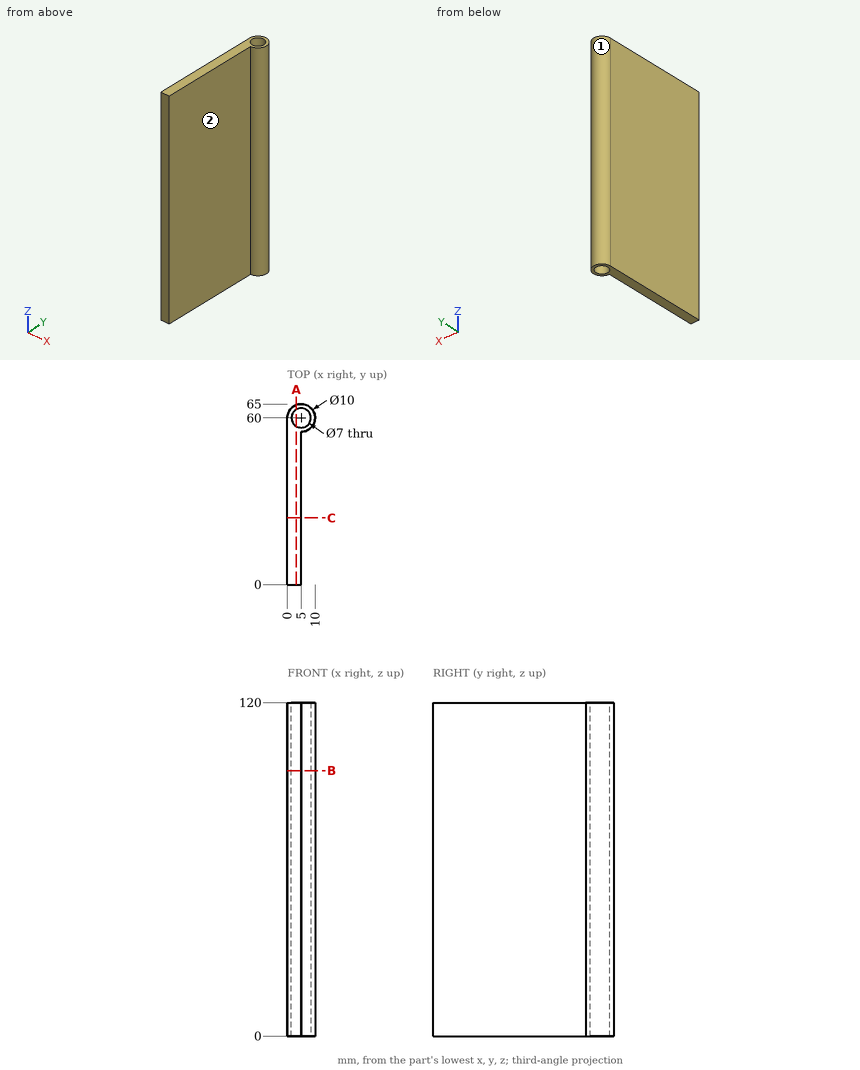
Could you check a few things on this drawing? It's one solid part, dimensions in mm from its lowest x, y, z. A direction names the side the tool comes from. Round coordinates to 2 decimals unless told otherwise and drop trailing zeros. Loops run counter-clockwise (first coordinate to the right, second up) from the corner with the lowest first, then second, coordinate; pieces in that order, holes last. Notation, with made-up numbers: M -29.5,77 L 27.5,77 A17 ccw 27.5,96 Z; hole C 0.5,-28.5 d1. An arc over 180 degrees is marked long. Write item = value, one per line. Start each with the question number.
(1) Which directions (+Z, -Z, +X, -X, +Y, -Y) give clear straight access to the entire face, cutting with the end or side of a thin tool? Please do the marked faces 1 and 2.
(2) I'm going to push a flat-ended pin straight in: P1, Ø6, axis at y = 10.5, z = 35.5, coming from the -X side. Where does the tip first touch, or does it pass through?
(3) Suppose I cut it at A-A on x = 3.25. Write out the boundary of the cut face in (y, z).
(4) Suppose I cut it at B-B on z = 95.5. Write out the boundary of the cut face in (x, y), plus the area to 3 significant figures.
(5) Suppose I cut it at C-C on y = 24. Write out the boundary of the cut face in (x, z).
(6) I need wall thicknesses on line 1 along X through (y, z) = (27.5, 15); line 2 along Y through (x, z) = (3.5, 64); line 3 along X through (y, z) = (62, 83). Which ranges of each line are inside material? Lowest first, please.
Answer block:
q1.face_1 = +Z, -Z
q1.face_2 = +Z, -Z, +X, -Y
q2.P1 = 0
q3.outline = M 0,0 L 56.97,0 L 56.97,120 L 0,120 Z; M 63.03,0 L 64.68,0 L 64.68,120 L 63.03,120 Z
q4.outline = M 0,0 L 5,0 L 5,55 A5 ccw long 0,60 Z; hole C 5,60 d7
q4.area = 320 mm²
q5.outline = M 0,0 L 5,0 L 5,120 L 0,120 Z
q6.line_1 = 0 to 5
q6.line_2 = 0 to 56.84, 63.16 to 64.77
q6.line_3 = 0.42 to 2.13, 7.87 to 9.58
